```python
from build123d import *

# Parameters (mm, degrees)
SKETCH_R        = 1.8
PAD_DEPTH       = 7
SKETCH001_R     = 2.9
POCKET_DEPTH    = 3
SKETCH002_W     = 13.4
SKETCH002_H     = 5
PAD001_DEPTH    = 6
SKETCH005_R     = 1.8
POCKET002_DEPTH = 5
PAD002_DEPTH    = 6
SKETCH009_W     = 8.2
SKETCH009_H     = 18
POCKET006_DEPTH = 9.6
POCKET003_DEPTH = 47.001
POCKET004_DEPTH = 5
POCKET005_DEPTH = 13.001
FILLET_R        = 1.5


with BuildPart() as part:
    # Sketch → Pad (new body)
    with BuildSketch(Plane.XY):
        with BuildLine():
            Line((-21.5, 0), (-21.5, -5))
            Line((-21.5, -5), (-8.1, -5))
            Line((-8.1, -5), (-8.1, -18))
            ThreePointArc((-10.421049, -20.922161), (-8.750867, -19.865898), (-8.1, -18))
            Line((-10.421049, -20.922161), (-22.018426, -23.616758))
            ThreePointArc((-22.018426, -23.616758), (-25.108802, -29.835142), (-18.415416, -31.683738))
            Line((-7.079536, -23.730259), (-18.415416, -31.683738))
            ThreePointArc((-7.079536, -23.730259), (-4.889394, -21.2293), (-4.1, -18))
            Line((-4.1, -18), (-4.1, -26))
            Line((-4.1, -26), (4.1, -26))
            Line((4.1, -18), (4.1, -26))
            ThreePointArc((4.1, -18), (4.889394, -21.2293), (7.079536, -23.730259))
            Line((7.079536, -23.730259), (18.415416, -31.683738))
            ThreePointArc((18.415416, -31.683738), (25.108802, -29.835142), (22.018426, -23.616758))
            Line((10.421049, -20.922161), (22.018426, -23.616758))
            ThreePointArc((8.1, -18), (8.750867, -19.865898), (10.421049, -20.922161))
            Line((8.1, -5), (8.1, -18))
            Line((21.5, -5), (8.1, -5))
            Line((21.5, -5), (21.5, 0))
            Line((21.5, 0), (4.1, 0))
            Line((4.1, 0), (4.1, -8))
            Line((-4.1, -8), (4.1, -8))
            Line((-4.1, 0), (-4.1, -8))
            Line((-21.5, 0), (-4.1, 0))
        make_face()
        with Locations((-21, -28)):
            Circle(SKETCH_R, mode=Mode.SUBTRACT)
        with Locations((21, -28)):
            Circle(SKETCH_R, mode=Mode.SUBTRACT)
    extrude(amount=PAD_DEPTH)

    # Sketch001 (on Face28 of Pad) → Pocket (cut)
    with BuildSketch(Plane.XY.offset(7)):
        with Locations((-21, -28)):
            Circle(SKETCH001_R)
        with Locations((21, -28)):
            Circle(SKETCH001_R)
    extrude(amount=-POCKET_DEPTH, mode=Mode.SUBTRACT)

    # Sketch002 (on Face5 of Pocket) → Pad001 (join)
    with BuildSketch(Plane.XY.offset(7)):
        with Locations((14.8, -2.5)):
            Rectangle(SKETCH002_W, SKETCH002_H)
        with Locations((-14.8, -2.5)):
            Rectangle(SKETCH002_W, SKETCH002_H)
    extrude(amount=PAD001_DEPTH)

    # Sketch005 (on Face32 of Pad001) → Pocket002 (cut)
    with BuildSketch(Plane(origin=(0, 0, 0), x_dir=(-1, 0, 0), z_dir=(0, 1, 0))):
        with Locations((-16, 9)):
            Circle(SKETCH005_R)
        with Locations((16, 9)):
            Circle(SKETCH005_R)
    extrude(amount=-POCKET002_DEPTH, mode=Mode.SUBTRACT)

    # Sketch003 (on Face3 of Pad001) → Pad002 (join)
    with BuildSketch(Plane.XY.offset(7)):
        Polygon((-8.1, -8), (-8.1, -18), (-4.1, -18), (-4.1, -26), (4.1, -26), (4.1, -18), (8.1, -18), (8.1, -8), align=None)
    extrude(amount=PAD002_DEPTH)

    # Sketch009 (on Face1 of Pad002) → Pocket006 (cut)
    with BuildSketch(Plane(origin=(0, 0, 0), x_dir=(1, 0, 0), z_dir=(0, 0, -1))):
        with Locations((0, 17)):
            Rectangle(SKETCH009_W, SKETCH009_H)
    extrude(amount=-POCKET006_DEPTH, mode=Mode.SUBTRACT)

    # Sketch006 → Pocket003 (cut, through all)
    with BuildSketch(Plane(origin=(-21.5, 0, 0), x_dir=(0, -1, 0), z_dir=(-1, 0, 0))):
        Polygon((5, 0), (0, 0), (0, 5), align=None)
    extrude(amount=-POCKET003_DEPTH, mode=Mode.SUBTRACT)

    # Sketch007 (on Face37 of Pocket003) → Pocket004 (cut)
    with BuildSketch(Plane.XZ.offset(5)):
        Polygon((-21.5, 0), (-21.5, 9), (-12.5, 0), align=None)
        Polygon((21.5, 0), (21.5, 9), (12.5, 0), align=None)
    extrude(amount=-POCKET004_DEPTH, mode=Mode.SUBTRACT)

    # Sketch008 (on Face18 of Pocket004) → Pocket005 (cut, through all)
    with BuildSketch(Plane.XY.offset(13)):
        with BuildLine():
            ThreePointArc((1.8, -14), (0, -12.2), (-1.8, -14))
            Line((-1.8, -14), (-1.8, -20))
            ThreePointArc((-1.8, -20), (0, -21.8), (1.8, -20))
            Line((1.8, -14), (1.8, -20))
        make_face()
    extrude(amount=-POCKET005_DEPTH, mode=Mode.SUBTRACT)

    # Fillet
    fillet_edges = [part.edges().sort_by_distance(p)[0] for p in [
        (12.747476, -27.706999, 0),
        (-12.747476, -27.706999, 0),
        (-12.747476, -27.706999, 7),
        (12.747476, -27.706999, 7),
    ]]
    fillet(fillet_edges, radius=FILLET_R)


solid = part.part
```
Design review of the part built by this model. Coordinates are the model's own, in mm. A direction names the side the tool comes from. Round coordinates to 2 decimals unless told otherwise and drop trailing zeros. Write each loop counter-clockwise with the first axis right and the second up, starting at its lowest first coordinate (ties: lowest second). Pieces come first, ordered by that corner, then holes.
Item 1: We need section D-D on y = -7.5. Write out the cut boundary in (x, z), and give its area (3 significant figures).
Item 2: The part is to be moulded in two halves that separate along X. For faces 4 (the flat face through (-19, -28, 4)), 5 (the flat face through (15, -2, 13)), 6 (the flat face through (16.14, -22.25, 3.47)), say which applies: +X half, -X half, draft (parallel to the pull), parting line (faces both ways), or undercut.
Item 3: We need section B-B on y = -17.5. Write out the cut boundary in (x, z), and give its area (3 significant figures).
Item 4: Clearance check with flat-ended pins moving along their axes: pin 1 Ø1.5 at (x, z) = (19.5, 4.5) entering from +Y; pin 2 Ø1.7 at (y, z) = (-23.5, 11) entering from +X; pin 3 Ø4.5 at (x, y) = (-21, -28) entering from -Z; pin 4 Ø3 at (x, z) = (-3, 11) entering from +Y. State where each tip first meets the part, or that it passes through.
Item 5: We need section A-A on z = 2.25. Write out the cut boundary in (x, y).
Item 6: For probe 1 along X at (y, z) = (-18.5, 12); probe 2 along X at (y, z) = (-28, 0.5); probe 3 along X at (y, z) = (-28, 2.85), list the stretches that pass through material, from the lowest coordinate up.
Item 7: We need section C-C on x = 0. Write out the cut boundary in (y, z).
Item 8: For faces 1 (the flat face through (1.8, -17, 11)), 2 (the flat face through (-16.14, -22.25, 3.47)), 3 (the cylindrical face through (7.65, -11.41, 0.43)), list the 3-axis set-ups (+Z, -Z, +X, -X, +Y, -Y) from which the entire face can be reached by the end or side of a thin tool; tool diameter is ignored.
Returned:
1. outline: (-8.1, 1.5) arc R1.5 ccw to (-6.6, 0) - (-5.6, 0) arc R1.5 ccw to (-4.1, 1.5) - (-4.1, 7) - (-8.1, 7) - close; (4.1, 1.5) arc R1.5 ccw to (5.6, 0) - (6.6, 0) arc R1.5 ccw to (8.1, 1.5) - (8.1, 7) - (4.1, 7) - close
1. area: 54.1 mm2
2. face 4: undercut
2. face 5: draft
2. face 6: +X half
3. outline: (-8.1, 1.5) arc R1.5 ccw to (-6.6, 0) - (-5.6, 0) arc R1.5 ccw to (-4.1, 1.5) - (-4.1, 9.6) - (-1.8, 9.6) - (-1.8, 13) - (-8.1, 13) - close; (1.8, 9.6) - (4.1, 9.6) - (4.1, 1.5) arc R1.5 ccw to (5.6, 0) - (6.6, 0) arc R1.5 ccw to (8.1, 1.5) - (8.1, 13) - (1.8, 13) - close
3. area: 118 mm2
4. pin 1: stops at y = -22.86
4. pin 2: stops at x = 4.1
4. pin 3: stops at z = 0
4. pin 4: stops at y = -8
5. outline: (-22.02, -23.62) arc R4.5 ccw (long way) to (-18.42, -31.68) - (-7.08, -23.73) arc R7 ccw to (-4.1, -18) - (-4.1, -2.75) - (-14.75, -2.75) - (-14.75, -5) - (-8.1, -5) - (-8.1, -18) arc R3 cw to (-10.42, -20.92) - close; (4.1, -18) arc R7 ccw to (7.08, -23.73) - (18.42, -31.68) arc R4.5 ccw (long way) to (22.02, -23.62) - (10.42, -20.92) arc R3 cw to (8.1, -18) - (8.1, -5) - (14.75, -5) - (14.75, -2.75) - (4.1, -2.75) - close; hole circle Ø3.6 at (-21, -28); hole circle Ø3.6 at (21, -28)
6. probe 1: x = -4.1 to -1.8, 1.8 to 4.1
6. probe 2: x = -25.12 to -22.8, -19.2 to -13.83, 13.83 to 19.2, 22.8 to 25.12
6. probe 3: x = -25.5 to -22.8, -19.2 to -13.17, 13.17 to 19.2, 22.8 to 25.5
7. outline: (-26, 9.6) - (-21.8, 9.6) - (-21.8, 13) - (-26, 13) - close; (-12.2, 9.6) - (-8, 9.6) - (-8, 13) - (-12.2, 13) - close
8. face 1: +Z, -Z
8. face 2: +Z, -Z, -X
8. face 3: -Z, +X
